Part model, mm, in its own coordinate system. Coordinates: 2 decimals unless noted, no trailing zeros. Loops run counter-clockwise (first coordinate to the right, second up) from the corner with the lowest first, then second, coordinate; pieces in that order, holes last. Notation, with made-up numbers: (4, 20.5) - (43, 20.5) arc R19 ccw to (43, 36.5) - close; hole circle Ø3 at (62, 67). An arc over 180 degrees is marked (long way). Answer as CSV lines item,"result".
from build123d import *

# Parameters (mm, degrees)
SKETCH1_R           = 2
BOSS_EXTRUDE1_DEPTH = 4


with BuildPart() as part:
    # Sketch1 → Boss-Extrude1 (new body)
    with BuildSketch(Plane(origin=(0, 0, 0), x_dir=(1, 0, 0), z_dir=(0, 1, 0))):
        with BuildLine():
            ThreePointArc((-5.220792314, 160), (0, 165.220792314), (5.220792314, 160))
            Line((5.220792314, 160), (5.220792314, 150))
            Line((5.220792314, 150), (150, 150))
            Line((150, 150), (150, -140.527151098))
            Line((150, -140.527151098), (160, -150.527151098))
            Line((160, -150.527151098), (170, -150.527151098))
            ThreePointArc((170, -150.527151098), (174.736424451, -155.263575549), (170, -160))
            Line((170, -160), (-170, -160))
            ThreePointArc((-170, -160), (-174.736424451, -155.263575549), (-170, -150.527151098))
            Line((-170, -150.527151098), (-160, -150.527151098))
            Line((-160, -150.527151098), (-150, -140.527151098))
            Line((-150, -140.527151098), (-150, 150))
            Line((-150, 150), (-5.220792314, 150))
            Line((-5.220792314, 150), (-5.220792314, 160))
        make_face()
        with Locations(Location((170, -155.263575549, 0), (0, 0, 270))):
            Circle(SKETCH1_R, mode=Mode.SUBTRACT)
        with Locations(Location((-170, -155.263575549, 0), (0, 0, 270))):
            Circle(SKETCH1_R, mode=Mode.SUBTRACT)
        with Locations(Location((0, 160, 0), (0, 0, 270))):
            Circle(SKETCH1_R, mode=Mode.SUBTRACT)
    extrude(amount=BOSS_EXTRUDE1_DEPTH)


solid = part.part
Q1. Saw through at B-B (z = -37.5). Give the cut face in (x, y).
Results:
outline,"(-150, 0) - (150, 0) - (150, 4) - (-150, 4) - close"
Q2. Saw through at A-A (y = 1.5). Give the cut face in (x, z).
Results:
outline,"(-170, 150.53) - (-160, 150.53) - (-150, 140.53) - (-150, -150) - (-5.22, -150) - (-5.22, -160) arc R5.22 ccw to (5.22, -160) - (5.22, -150) - (150, -150) - (150, 140.53) - (160, 150.53) - (170, 150.53) arc R4.74 ccw to (170, 160) - (-170, 160) arc R4.74 ccw to start; hole circle Ø4 at (-170, 155.26); hole circle Ø4 at (0, -160); hole circle Ø4 at (170, 155.26)"
Q3. Wall check: L1, parallel to Z at x = 170, y = 1.6; L2, parallel to X at y = 0.95, z = -39.5; L3, parallel to X at y = 1.65, z = -160. Give the ranges that are in metal, low to high.
Results:
L1,"z = 150.53 to 153.26, 157.26 to 160"
L2,"x = -150 to 150"
L3,"x = -5.22 to -2, 2 to 5.22"
Q4. Flat gauge pins, fed straight in: pin 1 (1.2 mm diameter, centred on x = 164.5, y = 1.5, fed in from -Z); pin 2 (3 mm diameter, centred on x = 170, z = 155.26, fed in from +Y); pin 3 (2 mm diameter, centred on x = -94.5, y = 2.5, fed in from -Z); pin 4 (2 mm diameter, centred on y = 1.5, z = -74.5, fed in from -X). Where does each tip first touch, or does it go through?
Results:
pin 1,"stops at z = 150.53"
pin 2,"passes through"
pin 3,"stops at z = -150"
pin 4,"stops at x = -150"
Q5. Saw through at C-C (x = -42.5). Give the cut face in (y, z), then the cut area to 3 significant figures.
Results:
outline,"(0, -150) - (4, -150) - (4, 160) - (0, 160) - close"
area,"1,240 mm^2"
Q6. Two-plate mould, pull along Z, no slides. Class faces 1 (the face through (2, 4, -5)), 2 (the face through (154.93, 1.972, 145.457)): released by +Z, released by -Z, zero draft, split by the parting line, or undercut.
Results:
face 1,"zero draft"
face 2,"released by -Z"
